The listing builds one solid part. Answer for the finished solid, in the listing's coordinates (mm). A direction names the side the tool comes from. Give positions to 0.01 mm unless a question says otherwise; leave off trailing zeros. Write each loop counter-clockwise with the first axis right and the second up, starting at its lowest first coordinate (ties: lowest second). Pieces come first, ordered by that corner, then holes.
```python
from build123d import *

# Parameters (mm, degrees)
BOSS_EXTRUDE2_DEPTH = 8
SHELL1_START        = 1
SHELL1_DEPTH        = 6
SKETCH5_W           = 6
SKETCH5_H           = 9.7
BOSS_EXTRUDE4_DEPTH = 1
FILLET1_R           = 2


# Read off the part's stored shape, not the designer's step: Shell1
with BuildPart() as part:
    # Sketch2 → Boss-Extrude2 (new body)
    with BuildSketch(Plane.XY):
        with BuildLine():
            Line((0, 20), (-32, 20))
            ThreePointArc((-32, 20), (-34.188489303, 19.649098779), (-36.157566157, 18.631575592))
            Line((-36.157566157, 18.631575592), (-38.071731179, 17.218424408))
            ThreePointArc((-38.071731179, 17.218424408), (-40.040808034, 16.200901221), (-42.229297337, 15.85))
            Line((-42.229297337, 15.85), (-70.229297337, 15.85))
            ThreePointArc((-70.229297337, 15.85), (-71.643510899, 15.264213562), (-72.229297337, 13.85))
            Line((-72.229297337, 13.85), (-72.229297337, 4.15))
            ThreePointArc((-72.229297337, 4.15), (-71.643510899, 2.735786438), (-70.229297337, 2.15))
            Line((-70.229297337, 2.15), (-42.229297337, 2.15))
            ThreePointArc((-42.229297337, 2.15), (-40.040808034, 1.799098779), (-38.071731179, 0.781575592))
            Line((-38.071731179, 0.781575592), (-36.157566157, -0.631575592))
            ThreePointArc((-36.157566157, -0.631575592), (-34.188489303, -1.649098779), (-32, -2))
            Line((-32, -2), (0, -2))
            ThreePointArc((0, -2), (1.414213562, -1.414213562), (2, 0))
            Line((2, 0), (2, 18))
            ThreePointArc((2, 18), (1.414213562, 19.414213562), (0, 20))
        make_face()
    extrude(amount=BOSS_EXTRUDE2_DEPTH)

    # Shell1 outline → Shell1 (cut)
    with BuildSketch(Plane.XY.offset(SHELL1_START)):
        with BuildLine():
            Line((-71.229297337, 13.85), (-72.229297337, 13.85))
            Line((-72.229297337, 13.85), (-72.229297337, 4.15))
            Line((-72.229297337, 4.15), (-71.229297337, 4.15))
            ThreePointArc((-71.229297337, 4.15), (-70.936404118, 3.442893219), (-70.229297337, 3.15))
            Line((-70.229297337, 3.15), (-42.229297337, 3.15))
            ThreePointArc((-42.229297337, 3.15), (-39.728166705, 2.748970033), (-37.477793157, 1.586086391))
            Line((-37.477793157, 1.586086391), (-35.563628135, 0.172935207))
            ThreePointArc((-35.563628135, 0.172935207), (-33.875847974, -0.699227525), (-32, -1))
            Line((-32, -1), (0, -1))
            ThreePointArc((0, -1), (0.707106781, -0.707106781), (1, 0))
            Line((1, 0), (1, 18))
            ThreePointArc((1, 18), (0.707106781, 18.707106781), (0, 19))
            Line((0, 19), (-32, 19))
            ThreePointArc((-32, 19), (-33.875847974, 18.699227525), (-35.563628135, 17.827064793))
            Line((-35.563628135, 17.827064793), (-37.477793157, 16.413913609))
            ThreePointArc((-37.477793157, 16.413913609), (-39.728166705, 15.251029967), (-42.229297337, 14.85))
            Line((-42.229297337, 14.85), (-70.229297337, 14.85))
            ThreePointArc((-70.229297337, 14.85), (-70.936404118, 14.557106781), (-71.229297337, 13.85))
        make_face()
    extrude(amount=SHELL1_DEPTH, mode=Mode.SUBTRACT)

    # Sketch5 → Boss-Extrude4 (add)
    with BuildSketch(Plane.ZY.offset(72.229297337)):
        with Locations((4, 9)):
            Rectangle(SKETCH5_W, SKETCH5_H)
    extrude(amount=-BOSS_EXTRUDE4_DEPTH)

    # Fillet1
    fillet1_edges = [part.edges().sort_by_distance(p)[0] for p in [
        (1.414213562, -1.414213562, 8),
        (2, 9, 8),
        (-37.114648668, 0.075, 0),
        (-40.040808034, 1.799098779, 0),
        (-56.229297337, 2.15, 0),
        (-71.643510899, 2.735786438, 0),
        (-72.229297337, 9, 0),
        (1.414213562, 19.414213562, 8),
        (-71.643510899, 15.264213562, 0),
        (-56.229297337, 15.85, 0),
        (-40.040808034, 16.200901221, 0),
        (-37.114648668, 17.925, 0),
        (-34.188489303, 19.649098779, 0),
        (-16, 20, 0),
        (1.414213562, 19.414213562, 0),
        (2, 9, 0),
        (-16, 20, 8),
        (1.414213562, -1.414213562, 0),
        (-16, -2, 0),
        (-34.188489303, -1.649098779, 0),
        (-34.188489303, 19.649098779, 8),
        (-37.114648668, 17.925, 8),
        (-40.040808034, 16.200901221, 8),
        (-56.229297337, 15.85, 8),
        (-71.643510899, 15.264213562, 8),
        (-72.229297337, 9, 8),
        (-34.188489303, -1.649098779, 8),
        (-71.643510899, 2.735786438, 8),
        (-56.229297337, 2.15, 8),
        (-40.040808034, 1.799098779, 8),
        (-37.114648668, 0.075, 8),
        (-16, -2, 8),
    ]]
    fillet(fillet1_edges, radius=FILLET1_R)


solid = part.part
```
Item 1: Consider probe 1 along Z at (x, y) = (-34, 3.25); probe 2 along Y at (x, z) = (-66.5, 2.25); probe 3 along X at (y, z) = (10, 4). Determine where each line is inside the solid, lowest interval first.
Conclusion:
probe 1: z = 0 to 1, 7 to 8
probe 2: y = 2.15 to 3.15, 14.85 to 15.85
probe 3: x = -72.23 to -71.23, 1 to 2
Item 2: Which of the six approach directions +Z, -Z, +X, -X, +Y, -Y give full straight-line access (tool end or side, diameter ignored) to faces 4 (the face through (-56, 15.85, 4)), 5 (the face through (-39.76, 2.76, 3.96)), 6 (the face through (-56.43, 15.28, 0.6))?
Conclusion:
face 4: +Z, -Z, -X, +Y
face 5: none
face 6: -Z, -X, +Y
Item 3: A cutting plane is placed at B-B, the plane y = 11.75. Give the vertices of the cut face in (x, z), plus the area to 3 significant figures.
Conclusion:
outline: (-72.23, 2) arc R2 ccw to (-70.23, 0) - (0, 0) arc R2 ccw to (2, 2) - (2, 6) arc R2 ccw to (0, 8) - (-70.23, 8) arc R2 ccw to (-72.23, 6) - close; hole (-71.23, 1) - (1, 1) - (1, 7) - (-71.23, 7) - close
area: 157 mm2
Item 4: Determine the mould class of faces 1 (the face through (-28, 9, 7)), 2 (the face through (-71.66, 2.75, 3.97)), 3 (the face through (-16.22, 19.43, 0.6)) for opening direction Z: pulls with the +Z half, pulls with the -Z half, needs draft (parallel to the pull), parting line crosses it, or undercut.
Conclusion:
face 1: undercut
face 2: needs draft
face 3: pulls with the -Z half
Item 5: A cutting plane is placed at A-A, the plane x = -45. Give the vertices of the cut face in (y, z), plus the area to 3 significant figures.
Conclusion:
outline: (2.15, 2) arc R2 ccw to (4.15, 0) - (13.85, 0) arc R2 ccw to (15.85, 2) - (15.85, 6) arc R2 ccw to (13.85, 8) - (4.15, 8) arc R2 ccw to (2.15, 6) - close; hole (3.15, 1) - (14.85, 1) - (14.85, 7) - (3.15, 7) - close
area: 36.0 mm2
Item 6: Each of these flat-tipped pins is pushed along its axis until it touches: P1, Ø1.5, axis at x = -38, y = 8.5, coming from the -Z side; P2, Ø4, axis at x = -51, z = 5, coming from the -Y side; P3, Ø4.5, axis at x = -51, z = 4.5, coming from the +Y side; P4, Ø1, axis at x = -46.5, y = 16, coming from the -Z side. Where does it stop, or does it pass through?
Conclusion:
P1: stops at z = 0
P2: stops at y = 2.15
P3: stops at y = 15.85
P4: stops at z = 0.87
